```python
from build123d import *


with BuildPart() as part:
    # Sketch1 → Revolve3 (revolve)
    with BuildSketch(Plane.XY, mode=Mode.PRIVATE) as revolve3_sk:
        with BuildLine():
            Line((-20.400236636, 14.424908344), (-20.400236636, -0.261393937))
            Line((-20.400236636, -0.261393937), (-21.719162522, -1.530451169))
            Line((-21.719162522, -1.530451169), (-22.980158849, -4.004592346))
            ThreePointArc((-22.980158849, -4.004592346), (-23.116228268, -4.502948705), (-23.042560909, -5.014267655))
            Line((-23.042560909, -5.014267655), (-22.653341709, -6.087520982))
            ThreePointArc((-22.653341709, -6.087520982), (-22.188474627, -6.694443039), (-21.459427679, -6.924543742))
            Line((-21.459427679, -6.924543742), (-19.4537368, -6.924543742))
            Line((-19.4537368, -6.924543742), (-20.15067284, -5.68654307))
            ThreePointArc((-20.15067284, -5.68654307), (-20.308987647, -5.1760969), (-20.243290857, -4.645717034))
            Line((-20.243290857, -4.645717034), (-19.985241777, -3.90500514))
            ThreePointArc((-19.985241777, -3.90500514), (-19.52155814, -3.287559507), (-18.785937053, -3.05281871))
            Line((-18.785937053, -3.05281871), (-16.386357218, -3.05281871))
            Line((-16.386357218, -3.05281871), (-16.386357218, 33.77718129))
            Line((-16.386357218, 33.77718129), (-29.06595701, 33.77718129))
            Line((-29.06595701, 33.77718129), (-29.06595701, 31.432997969))
            ThreePointArc((-29.06595701, 31.432997969), (-28.454196627, 29.779670421), (-26.91360112, 28.922752554))
            Line((-26.91360112, 28.922752554), (-22.552592527, 28.249304737))
            ThreePointArc((-22.552592527, 28.249304737), (-21.01199702, 27.39238687), (-20.400236636, 25.739059322))
            Line((-20.400236636, 25.739059322), (-20.400236636, 14.424908344))
        make_face()
    revolve(revolve3_sk.sketch.rotate(Axis((-16.386357218, -3.05281871, 0), (0, 1, 0)), 270), axis=Axis((-16.386357218, -3.05281871, 0), (0, 1, 0)))


solid = part.part
```
The listing builds one solid part. Answer for the finished solid, in the listing's coordinates (mm). A direction names the side the tool comes from. Coordinates: 2 decimals unless noted, no trailing zeros. Order: outer loops, then holes, each group sorted by start corner. A loop starts at its lowest first (then second) coordinate and runs counter-clockwise, first axis right, second up. Notation, with made-up numbers: M 36,-25 L 47,-25 A8 ccw 47,-21 Z; hole C 31,-35 d8. An arc over 180 degrees is marked long. Answer as a JSON object with one key per item and string values. Group by question number.
1. Section B-B on y = 17.5 is taken. Write down the section's boundary in (x, z), then the cut area to 3 significant figures.
2. Straight lines are drawn through the part: line 1 (Y direction, x = -21, z = 0.5); line 2 (Z direction, x = -20, y = 10); line 3 (X direction, y = 12, z = 1). For each, find the intervals that lie inside material, in ascending order.
3. A tool of negligible diameter and unlimited length cuts with its end or side. For faces 1 (the cylindrical face through (-28.96, 32.59, 1.65)), 2 (the conical face through (-20.95, -1.69, -2.91)), from which of +Z, -Z, +X, -X, +Y, -Y can it reach the whole face along a straight path? Write none if from no direction.
4. Flat-ended cylindrical pins translate along their axes: P1, Ø1.5, axis at x = -23, y = 11, coming from the +Z side; P2, Ø1, axis at x = -16, y = 2.5, coming from the -Z side; P3, Ø10, axis at x = -17, y = 1.5, coming from the +Z side; P4, Ø6, axis at y = 23.5, z = 0.5, coming from the +X side. Find the tip coordinate at first contact, or state that the pin passes through.
5. Determine the mould class of faces 3 (the flat face through (-17, 33.777, 0)), 4 (the flat face through (-16, -3.053, 0)), 5 (the cylindrical face through (-12.825, 12.557, -1.852)) for opening direction Z: released by +Z, released by -Z, zero draft, split by the parting line, or undercut.
Values follow:
{
 "1": {"outline": "C -16.39,0 d8.03", "area": "50.6 mm2"},
 "2": {"line 1": "-6.92 to -0.86, 27.41 to 33.78", "line 2": "-1.75 to 1.75", "line 3": "-20.27 to -12.5"},
 "3": {"face 1": "+Y, -Y", "face 2": "none"},
 "4": {"P1": "through", "P2": "z = -4.01", "P3": "z = 6.32", "P4": "x = -12.26"},
 "5": {"face 3": "zero draft", "face 4": "undercut", "face 5": "split by the parting line"}
}
